Input: part model. Units: mm. Frame: model coordinates. A direction names the side the tool comes from. Give positions to 0.01 mm unless a question says otherwise; leave off trailing zeros. Loops run counter-clockwise (first coordinate to the right, second up) from the corner with the lowest first, then second, coordinate; pieces in that order, holes last. Notation, with made-up numbers: M 89,-35 L 105,-35 A17 cw 105,-7 Z; hole C 1.5,18 d6. An arc over 180 degrees is marked long. Use CSV: the item, a comma, the result in double quotes. Start each with the question number.
Q1. Section B-B, the plane y = -1.3. Output: boundary loops of the cut face in (x, z) (3 decimals), plus the area to 3 significant figures.
Q2. Section A-A, the plane z = -16.5. Output: boundary loops of the cut face in (x, y), plus the area to 3 significant figures.
Q3. Section C-C, the plane x = -24.5. Output: boundary loops of the cut face in (y, z), plus the area to 3 significant figures.
Q4. Pull-direction query (X, two-part tool) for faces 6 (the flat face through (26, 0, -6.646)), 7 (the flat face through (-7.916, 0, -17)), 8 (the flat face through (-23.749, 0, 13)); classes: released by +X, released by -X, zero draft, split by the parting line, or undercut.
Q5. Section D-D, the plane z = 10.5. Output: boundary loops of the cut face in (x, y).
Q6. Material intervals for line 1 along Z through (x, y) = (26, -2.4); line 2 along Z through (x, y) = (4, 2.2) (3 decimals); line 3 along X through (y, z) = (-1.2, 15), sorted ascending.
Q7. Reachability of faces 1 (the flat face through (-26, 0, 6.646)), 2 (the flat face through (7.916, 0, -17)), 3 (the flat face through (23.749, 0, -13)), 4 (the flat face through (-26, 0, -6.646)), 5 (the flat face through (26, 0, 6.646)) from +Z, -Z, +X, -X, +Y, -Y: full face, straight path, thin tool, end or side. Return the list, or none.
Q8. Pin query (flat end, axial travel): pin 1 (2.5 mm diameter, centred on y = 1.5, z = -16.5, fed in from +X); pin 2 (2.5 mm diameter, centred on x = -27, y = -0.5, fed in from +Z); pin 3 (1.6 mm diameter, centred on y = 0, z = -17, fed in from -X). Return the tip coordinate at first contact, or that it passes through.
from build123d import *

# Parameters (mm, degrees)
SKETCH21_W          = 47.498
SKETCH21_H          = 39.878
BOSS_EXTRUDE1_DEPTH = 2.667
SKETCH22_W          = 5.334
SKETCH22_H          = 13.292666666
BOSS_EXTRUDE2_DEPTH = 5.334
CAVITY1_START       = -19.939
CAVITY1_OUTLINE_W   = 15.832666666
CAVITY1_OUTLINE_H   = 5.334
CAVITY1_DEPTH       = 5.334


# Read off the part's stored shape, not the designer's step: Cavity1
with BuildPart() as part:
    # Sketch21 → Boss-Extrude1 (new, symmetric)
    with BuildSketch(Plane(origin=(0, 0, 0), x_dir=(1, 0, 0), z_dir=(0, 1, 0))):
        Rectangle(SKETCH21_W, SKETCH21_H)
    extrude(amount=BOSS_EXTRUDE1_DEPTH, both=True)

    # Sketch22 → Boss-Extrude2 (add, through all)
    with BuildSketch(Plane(origin=(0, 2.667, 0), x_dir=(-1, 0, 0), z_dir=(0, 1, 0))):
        with Locations((26.416, 0)):
            Rectangle(SKETCH22_W, SKETCH22_H)
        with Locations((-26.416, 0)):
            Rectangle(SKETCH22_W, SKETCH22_H)
    extrude(amount=-BOSS_EXTRUDE2_DEPTH)

    # Cavity1 outline → Cavity1 (cut)
    with BuildSketch(Plane.XY.offset(CAVITY1_START)):
        Rectangle(CAVITY1_OUTLINE_W, CAVITY1_OUTLINE_H)
    extrude(amount=CAVITY1_DEPTH, mode=Mode.SUBTRACT)


solid = part.part
A:
1,outline,"M -29.083,-6.646 L -23.749,-6.646 L -23.749,-19.939 L -7.916,-19.939 L -7.916,-14.605 L 7.916,-14.605 L 7.916,-19.939 L 23.749,-19.939 L 23.749,-6.646 L 29.083,-6.646 L 29.083,6.646 L 23.749,6.646 L 23.749,19.939 L -23.749,19.939 L -23.749,6.646 L -29.083,6.646 Z"
1,area,"1,950 mm^2"
2,outline,"M -23.75,-2.67 L -7.92,-2.67 L -7.92,2.67 L -23.75,2.67 Z; M 7.92,-2.67 L 23.75,-2.67 L 23.75,2.67 L 7.92,2.67 Z"
2,area,"169 mm^2"
3,outline,"M -2.67,-6.65 L 2.67,-6.65 L 2.67,6.65 L -2.67,6.65 Z"
3,area,"70.9 mm^2"
4,face 6,"zero draft"
4,face 7,"undercut"
4,face 8,"released by -X"
5,outline,"M -23.75,-2.67 L 23.75,-2.67 L 23.75,2.67 L -23.75,2.67 Z"
6,line 1,"-6.65 to 6.65"
6,line 2,"-14.605 to 19.939"
6,line 3,"-23.75 to 23.75"
7,face 1,"+Z, -X, +Y, -Y"
7,face 2,"-Z, +Y, -Y"
7,face 3,"-Z, +X, +Y, -Y"
7,face 4,"-Z, -X, +Y, -Y"
7,face 5,"+Z, +X, +Y, -Y"
8,pin 1,"x = 23.75"
8,pin 2,"z = 6.65"
8,pin 3,"x = -23.75"
